The listing builds one solid part. Answer for the finished solid, in the listing's coordinates (mm). Face numbers are marked on the shaded views. A direction names the side the tool comes from. Round coordinates to 2 decimals unless told otherwise and drop trailing zeros. Loops run counter-clockwise (first coordinate to the right, second up) from the corner with the lowest first, then second, coordinate; pieces in that order, holes last. Notation, with made-up numbers: (68.5, 11.25) - (102.5, 11.25) arc R5 ccw to (102.5, 16.25) - close; hole circle Ø1 at (-33.5, -34). An arc over 180 degrees is marked (long way). One line per item, written item: value.
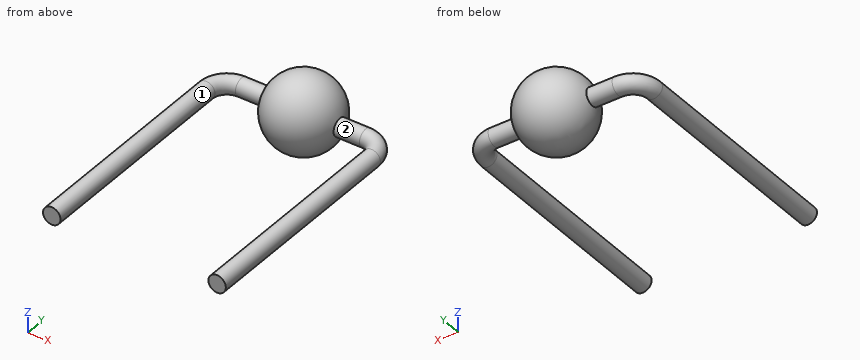
```python
from build123d import *

# Parameters (mm, degrees)
SKETCH_3_R = 0.423054932


with BuildPart() as part:
    # Эскиз1 → Повернуть2 (revolve)
    with BuildSketch(Plane(origin=(0, 0, 0), x_dir=(1, 0, 0), z_dir=(0, 1, 0))):
        with BuildLine():
            ThreePointArc((-1.749578385, 0.423054932), (0, 1.8), (1.749578385, 0.423054932))
            Line((1.749578385, 0.423054932), (1.749578385, 0))
            Line((1.749578385, 0), (-1.749578385, 0))
            Line((-1.749578385, 0), (-1.749578385, 0.423054932))
        make_face()
    revolve(axis=Axis((-29.751182373, 0, 0), (1, 0, 0)))

    # По траектории1: sweep along a path in Эскиз2
    with BuildLine(Plane.XY) as sweep_1_path:
        Line((0, 0), (-3, 0))
        ThreePointArc((-3, 0), (-3.707106781, -0.292893219), (-4, -1))
        Line((-4, -1), (-4, -11.514871198))
    # Эскиз3 → По траектории1 (sweep)
    with BuildSketch(Plane.ZY.offset(1.749578385)):
        Circle(SKETCH_3_R)
    sweep_1 = sweep(path=sweep_1_path.line)

    # Зеркальное отражение1: По траектории1 across plane
    add(sweep_1.mirror(Plane(origin=(0, 0, 0), x_dir=(0, 0, 1), z_dir=(1, 0, 0))))


solid = part.part
```
1) Each of these flat-tipped pins is pushed along its axis until it touches: pin 1 Ø2 at (x, y) = (-1.5, -7) entering from -Z; pin 2 Ø2 at (x, z) = (-2, -0.5) entering from -Y. Where does it stop, or does it pass through?
Final values:
pin 1: through
pin 2: y = -1.45
2) A cutting plane is placed at D-D on x = -2.5. Give the vertices of the cut face in (y, z).
Final values:
outline: circle Ø0.85 at (0, 0)
3) A cutting plane is placed at A-A on y = -4.5. Give the vertices of the cut face in (x, z).
Final values:
outline: circle Ø0.85 at (-4, 0); circle Ø0.85 at (4, 0)
4) For the marked faces 1 and 2, determine the directions among +Z, -Z, +X, -X, +Y, -Y from which every point of the face is accessible in a straight line to the end or side of a thin tool.
Final values:
face 1: -Y
face 2: none
5) Consider L1, parallel to X at y = -7.25, z = -0.15; L2, parallel to Z at x = 4, y = -2.25; L3, parallel to Y at x = -0.5, z = 0.25. Determine where each line is inside the solid, lowest interval first.
Final values:
L1: -4.4 to -3.6, 3.6 to 4.4
L2: -0.42 to 0.42
L3: -1.71 to 1.71
6) A cutting plane is placed at C-C on x = 0. Give the vertices of the cut face in (y, z), and give its area (3 significant figures).
Final values:
outline: circle Ø3.6 at (0, 0)
area: 10.2 mm2
7) A cutting plane is placed at B-B on z = 0. Give the vertices of the cut face in (x, y), and give its area (3 significant figures).
Final values:
outline: (-4.42, -11.51) - (-3.58, -11.51) - (-3.58, -1) arc R0.58 cw to (-3, -0.42) - (-1.75, -0.42) arc R1.8 ccw to (1.75, -0.42) - (3, -0.42) arc R0.58 cw to (3.58, -1) - (3.58, -11.51) - (4.42, -11.51) - (4.42, -1) arc R1.42 ccw to (3, 0.42) - (1.75, 0.42) arc R1.8 ccw to (-1.75, 0.42) - (-3, 0.42) arc R1.42 ccw to (-4.42, -1) - close
area: 32.7 mm2
